```python
from build123d import *

# Parameters (mm, degrees)
SKETCH1_R           = 40
SKETCH1_R_2         = 31
SKETCH1_W           = 7.7
SKETCH1_H           = 1.7
SKETCH1_W_2         = 1.7
SKETCH1_H_2         = 7.7
BOSS_EXTRUDE4_DEPTH = 1.5
SKETCH2_R           = 1.4
CUT_EXTRUDE2_DEPTH  = 1.5
CIRPATTERN3_COUNT   = 48


with BuildPart() as part:
    # Sketch1 → Boss-Extrude4 (new body)
    with BuildSketch(Plane(origin=(0, 0, 0), x_dir=(0, 0, -1), z_dir=(1, 0, 0))):
        Circle(SKETCH1_R)
        Circle(SKETCH1_R_2, mode=Mode.SUBTRACT)
        with Locations((0, 34)):
            Rectangle(SKETCH1_W, SKETCH1_H, mode=Mode.SUBTRACT)
        with Locations((34, 0)):
            Rectangle(SKETCH1_W_2, SKETCH1_H_2, mode=Mode.SUBTRACT)
        with Locations((0, -34)):
            Rectangle(SKETCH1_W, SKETCH1_H, mode=Mode.SUBTRACT)
        with Locations((-34, 0)):
            Rectangle(SKETCH1_W_2, SKETCH1_H_2, mode=Mode.SUBTRACT)
    extrude(amount=BOSS_EXTRUDE4_DEPTH)

    # Sketch2 → Cut-Extrude2 (cut)
    with BuildSketch(Plane(origin=(1.5, 0, 0), x_dir=(0, 0, -1), z_dir=(1, 0, 0))):
        with Locations((0, 37.5)):
            Circle(SKETCH2_R)
    cut_extrude2 = extrude(amount=-CUT_EXTRUDE2_DEPTH, mode=Mode.SUBTRACT)

    # CirPattern3: Cut-Extrude2 ×48 about axis
    cirpattern3_axis = Axis((0, 0, 0), (1, 0, 0))
    for i in range(1, CIRPATTERN3_COUNT):
        add(cut_extrude2.rotate(cirpattern3_axis, i * 360 / CIRPATTERN3_COUNT), mode=Mode.SUBTRACT)


solid = part.part
```
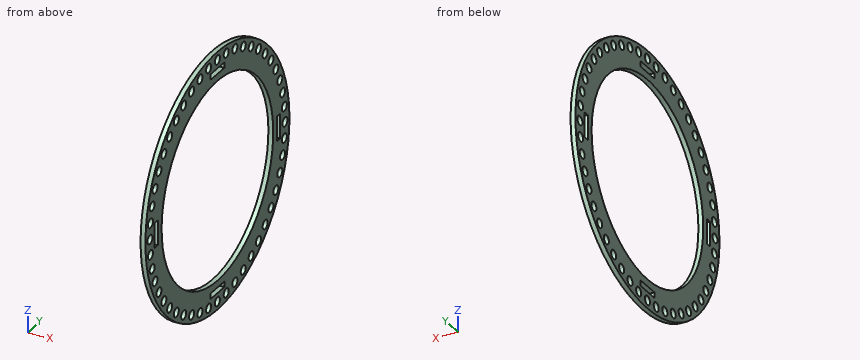
Input: part model. Units: mm. Frame: model coordinates. Give positions to 0.01 mm unless a question says otherwise; leave off trailing zeros. Order: outer loops, then holes, each group sorted by start corner. A loop starts at its lowest first (then second) coordinate and runs counter-clockwise, first axis right, second up. Notation, with made-up numbers: (56, 22.5) - (67, 22.5) arc R24 cw to (67, 48.5) - close; hole circle Ø2 at (74.25, 2). An arc over 180 degrees is marked (long way). Put each result on its own line as item: value.
Item 1: Contact query for a flat-ended pin moving along its axis: pin 1 (3.5 mm diameter, centred on y = 4.89, z = 37.18, fed in from +X). Output: stop coordinate, or through.
Found:
pin 1: stops at x = 1.5
Item 2: Section query C-C, the plane z = -18.75. Return loops of the section in (x, y).
Found:
outline: (0, -35.33) - (1.5, -35.33) - (1.5, -33.88) - (0, -33.88) - close; (0, -31.08) - (1.5, -31.08) - (1.5, -24.69) - (0, -24.69) - close; (0, 24.69) - (1.5, 24.69) - (1.5, 31.08) - (0, 31.08) - close; (0, 33.88) - (1.5, 33.88) - (1.5, 35.33) - (0, 35.33) - close
Item 3: Section query A-A, the plane z = 0. Return loops of the section in (x, y), then the cut area to 3 significant figures.
Found:
outline: (0, -40) - (1.5, -40) - (1.5, -38.9) - (0, -38.9) - close; (0, -36.1) - (1.5, -36.1) - (1.5, -34.85) - (0, -34.85) - close; (0, -33.15) - (1.5, -33.15) - (1.5, -31) - (0, -31) - close; (0, 31) - (1.5, 31) - (1.5, 33.15) - (0, 33.15) - close; (0, 34.85) - (1.5, 34.85) - (1.5, 36.1) - (0, 36.1) - close; (0, 38.9) - (1.5, 38.9) - (1.5, 40) - (0, 40) - close
area: 13.5 mm^2
Item 4: Ray query, L1, parallel to Y at x = 0.55, z = -2; L2, parallel to Y at x = 0.25, z = -14.5; L3, parallel to Z at x = 0.35, y = -18. Return the intervals inside material, ascending. Write a range as from..to.
Found:
L1: y = -39.95..-34.85, -33.15..-30.94, 30.94..33.15, 34.85..39.95
L2: y = -37.28..-36.04, -33.25..-27.4, 27.4..33.25, 36.04..37.28
L3: z = -35.72..-33.66, -31.29..-25.24, 25.24..31.29, 33.66..35.72
